from build123d import *

# Parameters (mm, degrees)
SKETCH1_W           = 304.8
SKETCH1_H           = 50.8
SKETCH1_W_2         = 5.9944
SKETCH1_H_2         = 12.7
BOSS_EXTRUDE1_DEPTH = 5.9944
SKETCH3_W           = 247.65
SKETCH3_H           = 1.4875
CUT_EXTRUDE3_DEPTH  = 6.9944
FILLET4_R           = 0.7
SKETCH4_W           = 28.575
SKETCH4_H           = 50.8
BOSS_EXTRUDE2_DEPTH = 5.9944
SKETCH5_W           = 5.9944
SKETCH5_H           = 12.7
CUT_EXTRUDE4_DEPTH  = 6.9944
FILLET5_R           = 3.175
CUT_EXTRUDE5_DEPTH  = 6.9944
SKETCH7_W           = 5.9944
SKETCH7_H           = 12.7
CUT_EXTRUDE6_DEPTH  = 6.9944


with BuildPart() as part:
    # Sketch1 → Boss-Extrude1 (new body)
    with BuildSketch(Plane.XY):
        with Locations((-152.4, 25.4)):
            Rectangle(SKETCH1_W, SKETCH1_H)
        with Locations((-15.6972, 12.7)):
            Rectangle(SKETCH1_W_2, SKETCH1_H_2, mode=Mode.SUBTRACT)
        with Locations((-15.6972, 38.1)):
            Rectangle(SKETCH1_W_2, SKETCH1_H_2, mode=Mode.SUBTRACT)
        with Locations((-257.3528, 38.1)):
            Rectangle(SKETCH1_W_2, SKETCH1_H_2, mode=Mode.SUBTRACT)
        with Locations((-257.3528, 12.7)):
            Rectangle(SKETCH1_W_2, SKETCH1_H_2, mode=Mode.SUBTRACT)
        with Locations((-295.4528, 12.7)):
            Rectangle(SKETCH1_W_2, SKETCH1_H_2, mode=Mode.SUBTRACT)
        with Locations((-295.4528, 38.1)):
            Rectangle(SKETCH1_W_2, SKETCH1_H_2, mode=Mode.SUBTRACT)
    extrude(amount=BOSS_EXTRUDE1_DEPTH)

    # Sketch3 → Cut-Extrude3 (cut, through all)
    with BuildSketch(Plane.XY.offset(5.9944)):
        with Locations((-136.525, 50.05625)):
            Rectangle(SKETCH3_W, SKETCH3_H)
        with Locations((-136.525, 0.74375)):
            Rectangle(SKETCH3_W, SKETCH3_H)
    extrude(amount=-CUT_EXTRUDE3_DEPTH, mode=Mode.SUBTRACT)

    # Fillet4
    fillet4_edges = [part.edges().sort_by_distance(p)[0] for p in [
        (-260.35, 49.3125, 2.9972),
        (-260.35, 50.8, 2.9972),
        (-12.7, 50.8, 2.9972),
        (-12.7, 49.3125, 2.9972),
        (-12.7, 0, 2.9972),
        (-260.35, 0, 2.9972),
        (-260.35, 1.4875, 2.9972),
        (-12.7, 1.4875, 2.9972),
    ]]
    fillet(fillet4_edges, radius=FILLET4_R)

    # Sketch4 → Boss-Extrude2 (add)
    with BuildSketch(Plane.XY.offset(5.9944)):
        with Locations((14.2875, 25.4)):
            Rectangle(SKETCH4_W, SKETCH4_H)
    extrude(amount=-BOSS_EXTRUDE2_DEPTH)

    # Sketch5 → Cut-Extrude4 (cut, through all)
    with BuildSketch(Plane.XY.offset(5.9944)):
        with Locations((21.893276, 38.1)):
            Rectangle(SKETCH5_W, SKETCH5_H)
        with Locations((21.893276, 12.7)):
            Rectangle(SKETCH5_W, SKETCH5_H)
    extrude(amount=-CUT_EXTRUDE4_DEPTH, mode=Mode.SUBTRACT)

    # Fillet5
    fillet5_edges = [part.edges().sort_by_distance(p)[0] for p in [
        (28.575, 50.8, 2.9972),
        (28.575, 0, 2.9972),
        (-304.8, 0, 2.9972),
        (-304.8, 50.8, 2.9972),
    ]]
    fillet(fillet5_edges, radius=FILLET5_R)

    # Sketch6 → Cut-Extrude5 (cut, through all)
    with BuildSketch(Plane.XY.offset(5.9944)):
        with BuildLine():
            Line((-123.825, 19.05), (-149.225, 19.05))
            ThreePointArc((-149.225, 19.05), (-155.575, 25.4), (-149.225, 31.75))
            Line((-149.225, 31.75), (-123.825, 31.75))
            ThreePointArc((-123.825, 31.75), (-117.475, 25.4), (-123.825, 19.05))
        make_face()
        with BuildLine():
            Line((-60.325, 19.05), (-85.725, 19.05))
            ThreePointArc((-85.725, 19.05), (-92.075, 25.4), (-85.725, 31.75))
            Line((-85.725, 31.75), (-60.325, 31.75))
            ThreePointArc((-60.325, 31.75), (-53.975, 25.4), (-60.325, 19.05))
        make_face()
        with BuildLine():
            Line((-187.325, 19.05), (-212.725, 19.05))
            ThreePointArc((-212.725, 19.05), (-219.075, 25.4), (-212.725, 31.75))
            Line((-212.725, 31.75), (-187.325, 31.75))
            ThreePointArc((-187.325, 31.75), (-180.975, 25.4), (-187.325, 19.05))
        make_face()
    extrude(amount=-CUT_EXTRUDE5_DEPTH, mode=Mode.SUBTRACT)

    # Sketch7 → Cut-Extrude6 (cut, through all)
    with BuildSketch(Plane.XY.offset(5.9944)):
        with Locations((-269.6972, 38.1)):
            Rectangle(SKETCH7_W, SKETCH7_H)
        with Locations((-3.3528, 38.1)):
            Rectangle(SKETCH7_W, SKETCH7_H)
        with Locations((-269.6972, 12.7)):
            Rectangle(SKETCH7_W, SKETCH7_H)
        with Locations((-3.3528, 12.7)):
            Rectangle(SKETCH7_W, SKETCH7_H)
    extrude(amount=-CUT_EXTRUDE6_DEPTH, mode=Mode.SUBTRACT)


solid = part.part
Can you work these out from the model? Positions are in its coordinate system, mm. A direction names the side the tool comes from. Give positions to 0.01 mm unless a question says otherwise; leave off trailing zeros. Order: outer loops, then holes, each group sorted by start corner. A loop starts at its lowest first (then second) coordinate and runs counter-clockwise, first axis right, second up. Notation, with made-up numbers: M 88.25,83 L 95.25,83 A28 ccw 95.25,102 Z; hole C 70.25,-14.5 d1. An arc over 180 degrees is marked long. Use one line per item in the form item = value. Start each with the question number.
Item 1: For faces 1 (the flat face through (-295, 6.35, 3)), 2 (the flat face through (-140, 14, 0)), which set-ups out of +Z, -Z, +X, -X, +Y, -Y let a thin tool reach every point of the face, with its end or its side?
Item 2: Will these pins go through, and if not, where does the flat tip stop? pin 1 Ø3 at (x, z) = (-213.5, 2) entering from +Y; pin 2 Ø4 at (x, y) = (-134, 29.5) entering from -Z; pin 3 Ø3 at (x, z) = (-45.5, 4.5) entering from -Y.
Item 3: If we section it at C-C (y = 40): Write out the boundary of the cut face in (x, z) (3 decimals).
Item 4: If we section it at B-B (y = 25.4): Write out the boundary of the cut face in (x, z) (3 decimals), then the cut area to 3 significant figures.
Item 5: If we section it at A-A (x = -80): Write out the boundary of the cut face in (y, z), then the cut area to 3 significant figures.
Item 6: If I drill on line 1 along X through (y, z) = (26, 5.4) (3 decimals); line 2 along Y through (x, z) = (-189, 0.3); line 3 along X through (y, z) = (30, 2.4) (1 decimal), over which ranges is the centre line in solid material (lowest first)?
Item 7: If we section it at D-D (z = 4.5): State how many separate pieces and enclosed holes the cut face has, then the cut area to 3 significant figures.
Item 8: We'd pull the mould along X, two halves only. Please class faces 3 (the cylindrical face through (-92.073, 25.26, 3.039)), 4 (the flat face through (6, 0, 3)): +X half, -X half, draft (parallel to the pull), parting line (faces both ways), or undercut.
Outcome:
q1.face_1 = +Z, -Z
q1.face_2 = -Z, +X, -X, +Y, -Y
q2.pin_1 = 49.31
q2.pin_2 = through
q2.pin_3 = 1.49
q3.outline = M -304.8,0 L -298.45,0 L -298.45,5.994 L -304.8,5.994 Z; M -292.456,0 L -272.694,0 L -272.694,5.994 L -292.456,5.994 Z; M -266.7,0 L -260.35,0 L -260.35,5.994 L -266.7,5.994 Z; M -254.356,0 L -18.694,0 L -18.694,5.994 L -254.356,5.994 Z; M -12.7,0 L -6.35,0 L -6.35,5.994 L -12.7,5.994 Z; M -0.356,0 L 18.896,0 L 18.896,5.994 L -0.356,5.994 Z; M 24.89,0 L 28.575,0 L 28.575,5.994 L 24.89,5.994 Z
q4.outline = M -304.8,0 L -219.075,0 L -219.075,5.994 L -304.8,5.994 Z; M -180.975,0 L -155.575,0 L -155.575,5.994 L -180.975,5.994 Z; M -117.475,0 L -92.075,0 L -92.075,5.994 L -117.475,5.994 Z; M -53.975,0 L 28.575,0 L 28.575,5.994 L -53.975,5.994 Z
q4.area = 1,310 mm2
q5.outline = M 1.49,0 L 19.05,0 L 19.05,5.99 L 1.49,5.99 Z; M 31.75,0 L 49.31,0 L 49.31,5.99 L 31.75,5.99 Z
q5.area = 211 mm2
q6.line_1 = -304.8 to -219.047, -181.003 to -155.547, -117.503 to -92.047, -54.003 to 28.575
q6.line_2 = 1.49 to 19.05, 31.75 to 49.31
q6.line_3 = -304.8 to -217.1, -182.9 to -153.6, -119.4 to -90.1, -55.9 to 28.6
q7.separate_pieces = 1
q7.enclosed_holes = 15
q7.area = 13,900 mm2
q8.face_3 = undercut
q8.face_4 = draft
